For this review, take the finished solid that the model builds, in its own axes (mm). A direction names the side the tool comes from. Coordinates: 2 decimals unless noted, no trailing zeros. Loops run counter-clockwise (first coordinate to the right, second up) from the corner with the lowest first, then second, coordinate; pieces in that order, holes last. Notation, with made-up numbers: (54.5, 55) -> (97.5, 55) arc R25 ccw to (97.5, 85) -> close; hole circle Ø9 at (-1, 21). An arc over 180 degrees is marked (long way). Answer in a Markdown table with one row per item.
from build123d import *

# Parameters (mm, degrees)
SKETCH2_W               = 40
SKETCH2_H               = 14
SKETCH2_R               = 4
BOSS_EXTRUDE_WALL_DEPTH = 25
SKETCH2_3_W             = 40
SKETCH2_3_H             = 8
SKETCH2_3_R             = 2.25
BOSS_EXTRUDE2_DEPTH     = 6
SKETCH3_W               = 20
SKETCH3_H               = 1.5
CUT_EXTRUDE1_DEPTH      = 36.355339059
SKETCH4_R               = 2.25
CUT_EXTRUDE2_DEPTH      = 39.845849199


with BuildPart() as part:
    # Sketch2 → Boss-Extrude_wall (new body)
    with BuildSketch(Plane(origin=(0, 0, 0), x_dir=(1, 0, 0), z_dir=(0, 1, 0))):
        Rectangle(SKETCH2_W, SKETCH2_H)
        with Locations(Location((0, 0, 0), (0, 0, 270))):
            Circle(SKETCH2_R, mode=Mode.SUBTRACT)
    extrude(amount=BOSS_EXTRUDE_WALL_DEPTH)

    # Sketch2_3 → Boss-Extrude2 (add)
    # profile 1 of 2: a face of its own
    with BuildSketch(Plane(origin=(0, 0, 0), x_dir=(1, 0, 0), z_dir=(0, 1, 0))):
        with Locations((0, -11)):
            Rectangle(SKETCH2_3_W, SKETCH2_3_H)
        with Locations(Location((-10, -11, 0), (0, 0, 270))):
            Circle(SKETCH2_3_R, mode=Mode.SUBTRACT)
        with Locations(Location((10, -11, 0), (0, 0, 270))):
            Circle(SKETCH2_3_R, mode=Mode.SUBTRACT)
    # profile 2 of 2: a face of its own
    with BuildSketch(Plane(origin=(0, 0, 0), x_dir=(1, 0, 0), z_dir=(0, 1, 0))):
        with Locations((0, 11)):
            Rectangle(SKETCH2_3_W, SKETCH2_3_H)
        with Locations(Location((-10, 11, 0), (0, 0, 270))):
            Circle(SKETCH2_3_R, mode=Mode.SUBTRACT)
        with Locations(Location((10, 11, 0), (0, 0, 270))):
            Circle(SKETCH2_3_R, mode=Mode.SUBTRACT)
    extrude(amount=BOSS_EXTRUDE2_DEPTH)

    # Sketch3 → Cut-Extrude1 (cut, through all)
    with BuildSketch(Plane(origin=(0, 25, 0), x_dir=(1, 0, 0), z_dir=(0, 1, 0))):
        with Locations((-10, 0)):
            Rectangle(SKETCH3_W, SKETCH3_H)
    extrude(amount=-CUT_EXTRUDE1_DEPTH, mode=Mode.SUBTRACT)

    # Sketch4 → Cut-Extrude2 (cut, through all)
    with BuildSketch(Plane.XY.offset(7)):
        with Locations((-16, 20.25)):
            Circle(SKETCH4_R)
        with Locations((-16, 10.75)):
            Circle(SKETCH4_R)
    extrude(amount=-CUT_EXTRUDE2_DEPTH, mode=Mode.SUBTRACT)


solid = part.part
Item 1: For faces 1 (the flat face through (-12, 13, -0.75)), 2 (the flat face through (0, 6, -11)), 3 (the flat face through (0, 6, 11)), list the 3-axis set-ups (+Z, -Z, +X, -X, +Y, -Y) from which the entire face can be reached by the end or side of a thin tool; tool diameter is ignored.
Worked answers:
| item | result |
|---|---|
| face 1 | -X, +Y, -Y |
| face 2 | -Z, +X, -X, +Y |
| face 3 | +Z, +X, -X, +Y |
Item 2: Take a section at B-B, the plane z = -11. State the section outline as (x, y) points, and give its area (3 significant figures).
Worked answers:
| item | result |
|---|---|
| outline | (-20, 0) -> (-12.25, 0) -> (-12.25, 6) -> (-20, 6) -> close; (-7.75, 0) -> (7.75, 0) -> (7.75, 6) -> (-7.75, 6) -> close; (12.25, 0) -> (20, 0) -> (20, 6) -> (12.25, 6) -> close |
| area | 186 mm² |
Item 3: Take a section at D-D, the plane x = 10. State the section outline as (y, z) points.
Worked answers:
| item | result |
|---|---|
| outline | (0, -15) -> (6, -15) -> (6, -13.25) -> (0, -13.25) -> close; (0, -8.75) -> (6, -8.75) -> (6, -7) -> (25, -7) -> (25, 7) -> (6, 7) -> (6, 8.75) -> (0, 8.75) -> close; (0, 13.25) -> (6, 13.25) -> (6, 15) -> (0, 15) -> close |
Item 4: Take a section at A-A, the plane x = -10. State the section outline as (y, z) points, and give its area (4 significant figures).
Worked answers:
| item | result |
|---|---|
| outline | (0, -15) -> (6, -15) -> (6, -13.25) -> (0, -13.25) -> close; (0, -8.75) -> (6, -8.75) -> (6, -7) -> (25, -7) -> (25, -0.75) -> (0, -0.75) -> close; (0, 0.75) -> (25, 0.75) -> (25, 7) -> (6, 7) -> (6, 8.75) -> (0, 8.75) -> close; (0, 13.25) -> (6, 13.25) -> (6, 15) -> (0, 15) -> close |
| area | 354.5 mm² |
Item 5: Take a section at C-C, the plane y = 20.25. State the section outline as (x, z) points.
Worked answers:
| item | result |
|---|---|
| outline | (-20, -7) -> (-18.25, -7) -> (-18.25, -0.75) -> (-20, -0.75) -> close; (-20, 0.75) -> (-18.25, 0.75) -> (-18.25, 7) -> (-20, 7) -> close; (-13.75, -7) -> (20, -7) -> (20, 7) -> (-13.75, 7) -> (-13.75, 0.75) -> (-3.93, 0.75) arc R4 cw (long way) to (-3.93, -0.75) -> (-13.75, -0.75) -> close |
Item 6: The part is to be moulded in two halves that separate along Z. For faces 4 (the cylindrical face through (4, 12, 0)), 5 (the cylindrical face through (-8.48, 2.96, -12.66)), 6 (the flat face through (0, 3, -15)), 7 (the flat face through (4.2, 0, -0.2)), say which applies: +Z half, -Z half, draft (parallel to the pull), parting line (faces both ways), or undercut.
Worked answers:
| item | result |
|---|---|
| face 4 | undercut |
| face 5 | undercut |
| face 6 | -Z half |
| face 7 | draft |
Item 7: For L1, parallel to X at y = 3.35, z = 11; L2, parallel to Z at x = 0, y = 22; L3, parallel to Y at x = -16, z = -2.25, list the stretches that pass through material, from the lowest coordinate up.
Worked answers:
| item | result |
|---|---|
| L1 | -20 to -12.25, -7.75 to 7.75, 12.25 to 20 |
| L2 | -7 to -4, 4 to 7 |
| L3 | 0 to 8.5, 13 to 18, 22.5 to 25 |
Item 8: Insertion check: pin 1 (5 mm diameter, centred on x = -10, z = -11, fed in from +Y); pin 2 (13 mm diameter, centred on x = -10.5, y = 14, fed in from +Z); pin 3 (10 mm diameter, centred on x = 2.5, y = 14, fed in from -Z); pin 4 (3.5 mm diameter, centred on x = 10, z = 11, fed in from +Y). Each pin has a flat end and moves straight along its axis. Give the tip position at first contact, or say it passes through.
Worked answers:
| item | result |
|---|---|
| pin 1 | y = 6 |
| pin 2 | z = 7 |
| pin 3 | z = -7 |
| pin 4 | through |
